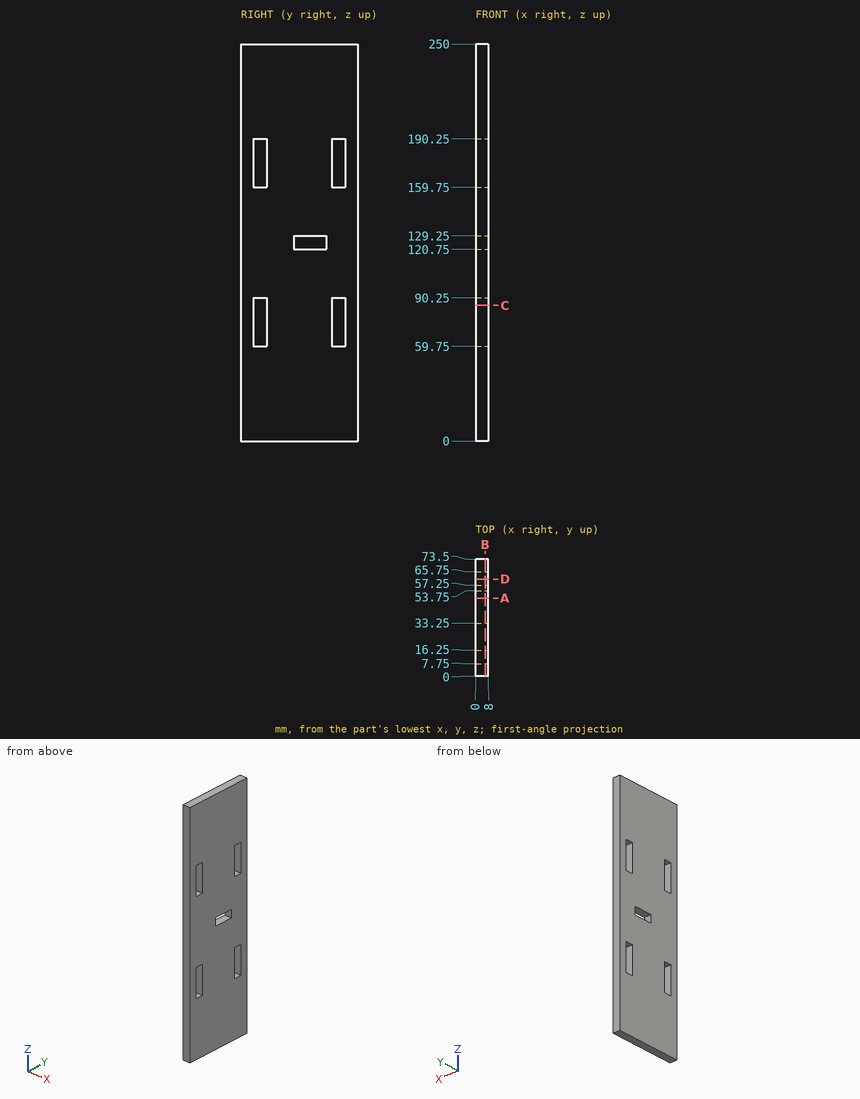
Part print with two shaded views. Sizes in mm from the minimum x, y, z corner. Give positions to 0.01 mm unless a question says otherwise; leave off trailing zeros. Order: outer loops, then holes, each group sorted by start corner. A loop starts at its lowest first (then second) coordinate and runs counter-clockwise, first axis right, second up. Notation, with made-up numbers: M 6,-6.5 L 35,-6.5 A5 cw 35,-0.5 Z; hole C 89,54 d11. An arc over 180 degrees is marked long. Put each result on its own line as item: value.
Item 1: Cut at D-D on y = 61. Write the cut outline in (x, z).
Results are:
outline: M 0,0 L 8,0 L 8,59.75 L 0,59.75 Z; M 0,90.25 L 8,90.25 L 8,159.75 L 0,159.75 Z; M 0,190.25 L 8,190.25 L 8,250 L 0,250 Z
Item 2: Cut at C-C on z = 85.5. Write the cut outline in (x, y).
Results are:
outline: M 0,0 L 8,0 L 8,7.75 L 0,7.75 Z; M 0,16.25 L 8,16.25 L 8,57.25 L 0,57.25 Z; M 0,65.75 L 8,65.75 L 8,73.5 L 0,73.5 Z
Item 3: Wall check: probe 1 along Y at (x, z) = (4.5, 79); probe 2 along Z at (x, y) = (2.25, 62). Give the ranges that are in metal, low to high.
Results are:
probe 1: 0 to 7.75, 16.25 to 57.25, 65.75 to 73.5
probe 2: 0 to 59.75, 90.25 to 159.75, 190.25 to 250
Item 4: Cut at B-B on x = 6. Write the cut outline in (y, z).
Results are:
outline: M 0,0 L 73.5,0 L 73.5,250 L 0,250 Z; hole M 7.75,59.75 L 16.25,59.75 L 16.25,90.25 L 7.75,90.25 Z; hole M 7.75,159.75 L 16.25,159.75 L 16.25,190.25 L 7.75,190.25 Z; hole M 33.25,120.75 L 53.75,120.75 L 53.75,129.25 L 33.25,129.25 Z; hole M 57.25,59.75 L 65.75,59.75 L 65.75,90.25 L 57.25,90.25 Z; hole M 57.25,159.75 L 65.75,159.75 L 65.75,190.25 L 57.25,190.25 Z
Item 5: Cut at A-A on y = 49. Write the cut outline in (x, z).
Results are:
outline: M 0,0 L 8,0 L 8,120.75 L 0,120.75 Z; M 0,129.25 L 8,129.25 L 8,250 L 0,250 Z
Item 6: Drop a flat-ended pin along its axis: pin 1 Ø2.5 at (x, z) = (5.5, 169.5) entering from -Y. Give the stop position or say it passes through.
Results are:
pin 1: y = 0
